```python
from build123d import *

# Parameters (mm, degrees)
SKETCH_1_W           = 89.86690944
SKETCH_1_H           = 19
EXTRUDE_1_DEPTH      = 2
SKETCH_2_W           = 2
SKETCH_2_H           = 12.5
EXTRUDE_2_DEPTH      = 6
EXTRUDE_3_DEPTH      = 3
SKETCH_4_W           = 2
SKETCH_4_H           = 6.25
REVOLVE_1_ANGLE      = 180
EXTRUDE_8_DEPTH      = 1.5
EXTRUDE_8_DEPTH_BACK = 3.5
SKETCH_11_W          = 9.25
SKETCH_11_H          = 3
SCALE_1_SCALE        = 1.6
CUT_EXTRUDE_START    = -2.4
SKETCH_13_W          = 14.8
SKETCH_13_H          = 4.8
CUT_EXTRUDE_3_DEPTH  = 2.4
SKETCH_16_W          = 2
SKETCH_16_H          = 2.2
CUT_EXTRUDE_5_DEPTH  = 4.8
EXTRUDE_START        = -3.190039
EXTRUDE_10_DEPTH     = 6.4
CUT_EXTRUDE_6_REACH  = 79.611
FILLET_1_R           = 2
SKETCH_19_W          = 20
SKETCH_19_H          = 15
EXTRUDE_11_DEPTH     = 3.2
FILLET_2_R           = 2


with BuildPart() as part:
    # 草图1 → 凸台-拉伸1 (new body)
    with BuildSketch(Plane.XY):
        Rectangle(SKETCH_1_W, SKETCH_1_H)
    extrude(amount=EXTRUDE_1_DEPTH)

    # 草图2 → 凸台-拉伸2 (add)
    with BuildSketch(Plane.XY.offset(2)):
        with Locations((32.68345472, 0)):
            Rectangle(SKETCH_2_W, SKETCH_2_H)
        with Locations((25.68345472, 0)):
            Rectangle(SKETCH_2_W, SKETCH_2_H)
        with Locations((18.68345472, 0)):
            Rectangle(SKETCH_2_W, SKETCH_2_H)
        with Locations((11.68345472, 0)):
            Rectangle(SKETCH_2_W, SKETCH_2_H)
        with Locations((4.68345472, 0)):
            Rectangle(SKETCH_2_W, SKETCH_2_H)
        with Locations((-2.31654528, 0)):
            Rectangle(SKETCH_2_W, SKETCH_2_H)
        with Locations((-9.31654528, 0)):
            Rectangle(SKETCH_2_W, SKETCH_2_H)
        with Locations((-16.31654528, 0)):
            Rectangle(SKETCH_2_W, SKETCH_2_H)
        with Locations((-23.31654528, 0)):
            Rectangle(SKETCH_2_W, SKETCH_2_H)
        with Locations((-30.31654528, 0)):
            Rectangle(SKETCH_2_W, SKETCH_2_H)
    extrude(amount=EXTRUDE_2_DEPTH)

    # 草图3 → 凸台-拉伸3 (add)
    with BuildSketch(Plane.XY.offset(2)):
        Polygon((-29.31654528, -2), (42.93345472, -2), (42.93345472, 2), (-36.31654528, 2), (-36.31654528, -2), align=None)
    extrude(amount=EXTRUDE_3_DEPTH)

    # 草图4 → 旋转1 (revolve)
    with BuildSketch(Plane.XY.offset(8)):
        with Locations((25.68345472, -3.125)):
            Rectangle(SKETCH_4_W, SKETCH_4_H)
        with Locations((32.68345472, -3.125)):
            Rectangle(SKETCH_4_W, SKETCH_4_H)
        with Locations((18.68345472, -3.125)):
            Rectangle(SKETCH_4_W, SKETCH_4_H)
        with Locations((11.68345472, -3.125)):
            Rectangle(SKETCH_4_W, SKETCH_4_H)
        with Locations((4.68345472, -3.125)):
            Rectangle(SKETCH_4_W, SKETCH_4_H)
        with Locations((-2.31654528, -3.125)):
            Rectangle(SKETCH_4_W, SKETCH_4_H)
        with Locations((-9.31654528, -3.125)):
            Rectangle(SKETCH_4_W, SKETCH_4_H)
        with Locations((-16.31654528, -3.125)):
            Rectangle(SKETCH_4_W, SKETCH_4_H)
        with Locations((-23.31654528, -3.125)):
            Rectangle(SKETCH_4_W, SKETCH_4_H)
        with Locations((-30.31654528, -3.125)):
            Rectangle(SKETCH_4_W, SKETCH_4_H)
    revolve(axis=Axis((-31.31654528, 0, 8), (-1, 0, 0)), revolution_arc=REVOLVE_1_ANGLE)

    # 草图11 → 凸台-拉伸8 (add, two sides: drawn at the far end of the back side and taken through both)
    with BuildSketch(Plane.XZ.offset(2).offset(-EXTRUDE_8_DEPTH_BACK)):
        with Locations((38.30845472, 3.5)):
            Rectangle(SKETCH_11_W, SKETCH_11_H)
    extrude(amount=EXTRUDE_8_DEPTH + EXTRUDE_8_DEPTH_BACK)


with BuildPart() as part_1:
    # 缩放比例1: scaled about (1.114528854, -0.016602301, 3.861170743)
    add(part.part.scale(SCALE_1_SCALE).moved(Location((-0.668717312, 0.009961381, -2.316702446))))

    # 草图13 → 切除-拉伸3 (cut)
    with BuildSketch(Plane.XZ.offset(5.59003862).offset(CUT_EXTRUDE_START)):
        with Locations((60.62481024, 3.283297554)):
            Rectangle(SKETCH_13_W, SKETCH_13_H)
    extrude(amount=CUT_EXTRUDE_3_DEPTH, mode=Mode.SUBTRACT)

    # 草图16 → 切除-拉伸5 (cut)
    with BuildSketch(Plane.XY.offset(5.683297554)):
        with Locations((67.02481024, -2.09003862)):
            Rectangle(SKETCH_16_W, SKETCH_16_H)
        with Locations((67.02481024, 2.10996138)):
            Rectangle(SKETCH_16_W, SKETCH_16_H)
    extrude(amount=-CUT_EXTRUDE_5_DEPTH, mode=Mode.SUBTRACT)

    # 草图17 → 凸台-拉伸10 (add)
    with BuildSketch(Plane(origin=(0, 0, 0), x_dir=(1, 0, 0), z_dir=(0, 1, 0)).offset(EXTRUDE_START)):
        with BuildLine():
            Line((-58.77518976, -5.683297554), (-58.77518976, -0.883297554))
            Line((-58.77518976, -0.883297554), (-67.445131169, -0.883297554))
            ThreePointArc((-67.445131169, -0.883297554), (-63.730184312, -4.40320806), (-58.77518976, -5.683297554))
        make_face()
    extrude(amount=EXTRUDE_10_DEPTH)

    # 草图18 → 切除-拉伸6 (cut, up to next)
    with BuildSketch(Plane(origin=(0, 3.20996138, 0), x_dir=(1, 0, 0), z_dir=(0, 1, 0)), mode=Mode.PRIVATE) as cut_extrude_6_sk1:
        with BuildLine():
            Line((-50.77518976, -3.283297554), (-59.153474578, -3.283297554))
            ThreePointArc((-59.153474578, -3.283297554), (-62.646552572, -2.664466304), (-65.714448246, -0.883297554))
            Line((-65.714448246, -0.883297554), (-67.445131169, -0.883297554))
            ThreePointArc((-67.445131169, -0.883297554), (-63.730184312, -4.40320806), (-58.77518976, -5.683297554))
            Line((-58.77518976, -5.683297554), (-50.77518976, -5.683297554))
            Line((-50.77518976, -5.683297554), (-50.77518976, -3.283297554))
        make_face()
    cut_extrude_6_tool1 = extrude(cut_extrude_6_sk1.sketch, amount=-CUT_EXTRUDE_6_REACH, mode=Mode.PRIVATE) & part_1.part
    add(cut_extrude_6_tool1.solids().sort_by_distance((-58.541843, 3.209961, 4.008165))[0], mode=Mode.SUBTRACT)

    # 圆角1
    fillet_1_edges = [part_1.edges().sort_by_distance(p)[0] for p in [
        (71.22481024, -15.190038619, -0.716702446),
        (-72.562244864, -15.190038619, -0.716702446),
        (-72.562244864, 15.209961381, -0.716702446),
        (71.22481024, 15.209961381, -0.716702446),
    ]]
    fillet(fillet_1_edges, radius=FILLET_1_R)

    # 草图19 → 凸台-拉伸11 (add)
    with BuildSketch(Plane(origin=(0, 0, -2.316702446), x_dir=(-1, 0, 0), z_dir=(0, 0, -1))):
        with Locations((-81.22481024, 0)):
            Rectangle(SKETCH_19_W, SKETCH_19_H)
        with Locations((82.562244864, 0)):
            Rectangle(SKETCH_19_W, SKETCH_19_H)
    extrude(amount=-EXTRUDE_11_DEPTH)

    # 圆角2
    fillet_2_edges = [part_1.edges().sort_by_distance(p)[0] for p in [
        (91.22481024, 7.5, -0.716702446),
        (91.22481024, -7.5, -0.716702446),
        (71.22481024, -7.5, -0.716702446),
        (71.22481024, 7.5, -0.716702446),
        (-92.562244864, -7.5, -0.716702446),
        (-92.562244864, 7.5, -0.716702446),
        (-72.562244864, 7.5, -0.716702446),
        (-72.562244864, -7.5, -0.716702446),
    ]]
    fillet(fillet_2_edges, radius=FILLET_2_R)


solid = part_1.part
```
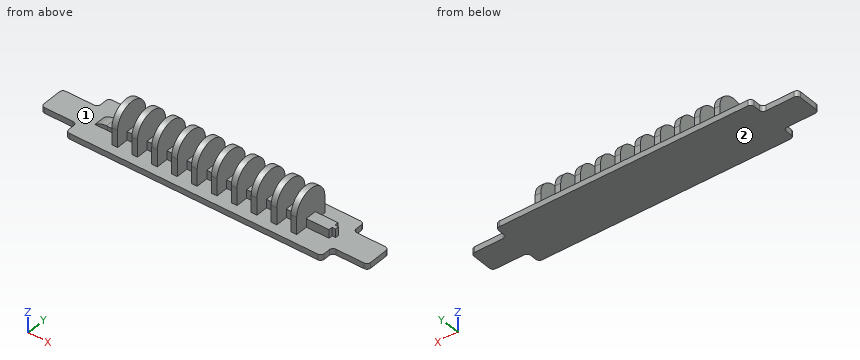
The model under review builds one solid part; all positions refer to its coordinate system, in mm. Face numbers are marked on the shaded views. Round coordinates to 2 decimals unless told otherwise and drop trailing zeros. Loops run counter-clockwise (first coordinate to the right, second up) from the corner with the lowest first, then second, coordinate; pieces in that order, holes last. Notation, with made-up numbers: M 42.5,14 L 55.5,14 A18 ccw 55.5,21 Z; hole C 33.25,65 d2. An arc over 180 degrees is marked long. Answer as a JSON object with one key per item and string values.
(1) Draft analysis for pull direction X (two halves, no side actions). For the marked faces 1 and 2, state which applies: released by +X, released by -X, zero draft, split by the parting line, or undercut.
Resolved:
{"face 1": "undercut", "face 2": "zero draft"}
(2) To check wall thickness, follow line 1 along Y through (x, z) = (-59, 3); line 2 along Z through (x, y) = (3.5, -12); line 3 along Z through (x, y) = (-18, -2.5). State the ranges of each line that lie inside material, in increasing order.
Resolved:
{"line 1": "-3.19 to 3.21", "line 2": "-2.32 to 0.88", "line 3": "-2.32 to 5.68"}
(3) Take a section at A-A on x = -23. Give the boundary of the cut face in (y, z).
Resolved:
{"outline": "M -15.19,-2.32 L 15.21,-2.32 L 15.21,0.88 L 3.21,0.88 L 3.21,5.68 L -3.19,5.68 L -3.19,0.88 L -15.19,0.88 Z"}
(4) Take a section at B-B on z = 16.5. Count the separate pieces of the cut face and the enclosed holes in it, and give its area (3 significant figures).
Resolved:
{"separate pieces": "10", "enclosed holes": "0", "area": "511 mm²"}
(5) Clearance check with flat-ended pins moving along their axes: P1, Ø3, axis at x = 0, y = -1, coming from the +Z side; P2, Ø4, axis at x = 23, z = 3.5, coming from the +Y side; P3, Ø3.5, axis at x = 51, z = 6.5, coming from the +Y side; P4, Ø15, axis at x = 17, y = -6.5, coming from the +Z side. State where each tip first meets the part, or that it passes through.
Resolved:
{"P1": "z = 5.68", "P2": "y = 3.21", "P3": "y = 10.01", "P4": "z = 20.48"}
